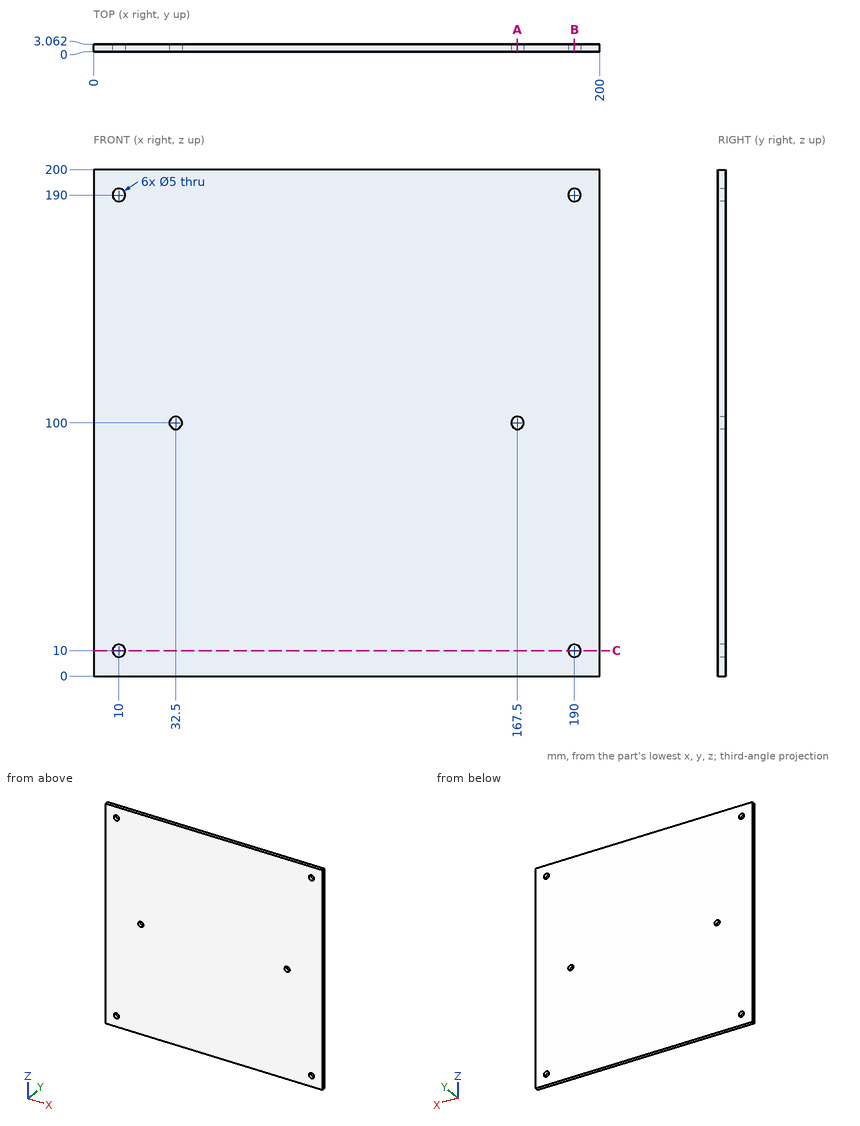
Study the drawing (mm; zero at the part's minimum x, y, z) and answer. Give positions to 0.01 mm unless a question says otherwise; leave off trailing zeros. Write each loop counter-clockwise with the first axis right and the second up, starting at its lowest first coordinate (ties: lowest second). Pieces come first, ordered by that corner, then holes.
(1) The part is cut by section C-C on z = 10. Write down the section's boundary in (x, y).
Final values:
outline: (0, 0) - (7.5, 0) - (7.5, 3.06) - (0, 3.06) - close; (12.5, 0) - (187.5, 0) - (187.5, 3.06) - (12.5, 3.06) - close; (192.5, 0) - (200, 0) - (200, 3.06) - (192.5, 3.06) - close
(2) The part is cut by section A-A on x = 167.5. Write down the section's boundary in (y, z).
Final values:
outline: (0, 0) - (3.06, 0) - (3.06, 97.5) - (0, 97.5) - close; (0, 102.5) - (3.06, 102.5) - (3.06, 200) - (0, 200) - close
(3) A flat-ended cylindrical pin translates along its axis: pin 1 Ø4.5 at (x, z) = (10, 10) entering from -Y. Find the tip coordinate at first contact, or state that the pin passes through.
Final values:
pin 1: passes through
(4) Straight lines are drawn through the part: line 1 (X direction, y = 0.85, z = 100); line 2 (X direction, y = 1.4, z = 10); line 3 (Z direction, x = 188, y = 2.2). For each, find the intervals that lie inside material, in ascending order.
Final values:
line 1: x = 0 to 30, 35 to 165, 170 to 200
line 2: x = 0 to 7.5, 12.5 to 187.5, 192.5 to 200
line 3: z = 0 to 8.5, 11.5 to 188.5, 191.5 to 200
(5) The part is cut by section B-B on x = 190. Write down the section's boundary in (y, z).
Final values:
outline: (0, 0) - (3.06, 0) - (3.06, 7.5) - (0, 7.5) - close; (0, 12.5) - (3.06, 12.5) - (3.06, 187.5) - (0, 187.5) - close; (0, 192.5) - (3.06, 192.5) - (3.06, 200) - (0, 200) - close
